For this review, take the finished solid that the model builds, in its own axes (mm). A direction names the side the tool comes from. Give positions to 0.01 mm unless a question says otherwise; leave off trailing zeros. Loops run counter-clockwise (first coordinate to the right, second up) from the corner with the lowest first, then second, coordinate; pieces in that order, holes last. Notation, with made-up numbers: (65, 4.5) - (119, 4.5) arc R13 cw to (119, 19.5) - close; hole circle Ø5 at (88.25, 14.5). An arc over 180 degrees is marked (long way). Use CSV: the item, a comma, the result in double quotes. Start each with the question number.
1. For faces 5 (the cylindrical face through (41.251, 19.965, 1.521)), 6 (the cylindrical face through (-43.94, 46.8, 4.14)), 7 (the flat face through (-49.85, 43.11, 11.9)), list the 3-axis set-ups (+Z, -Z, +X, -X, +Y, -Y) from which the entire face can be reached by the end or side of a thin tool; tool diameter is ignored.
2. Take a section at B-B on z = 10. State how many separate pieces and enclosed holes the cut face has, plus the area to 3 significant figures.
3. Wall thickness on line 1 (Y direction, x = 0, z = 2); line 2 (Z direction, x = 76, y = 23); line 3 (X direction, y = 18.5, z = 13.5): over which ranges is each line inside the solid? List them lowest first.
4. Mouldability with a two-part tool opening along Y and no side actions: class faces 1 (the flat face through (-47, 44, 24)), 2 (the cylindrical face through (40.62, 42.5, 1.52)), 3 (the flat face through (2.524, 54.735, 12.673)), 4 (the cylindrical face through (-51.829, 43.084, 4.141)) as pulls with the +Y half, pulls with the -Y half, needs draft (parallel to the pull), parting line crosses it, or undercut.
5. Take a section at A-A on y = 34. Give the boundary of the cut face in (x, z), plus the area to 3 significant figures.
6. Take a section at C-C on x = 20.5. Give the boundary of the cut face in (y, z), plus the area to 3 significant figures.
7. For pin 1 (3 mm diameter, centred on x = 50.5, z = 17, fed in from -Y); pin 2 (0.9 mm diameter, centred on x = -60, z = 1.5, fed in from +Y); pin 3 (3.5 mm diameter, centred on x = 14.5, z = 2, fed in from +Y), all flat-tipped, find the tip position at first contact; note any pin that passes through.
```python
from build123d import *

# Parameters (mm, degrees)
BOSS_EXTRUDE1_DEPTH = 3
BOSS_EXTRUDE2_DEPTH = 21
SKETCH3_R           = 1.5875
CUT_EXTRUDE1_DEPTH  = 111.972114009
FILLET3_R           = 4
FILLET4_R           = 4


with BuildPart() as part:
    # Sketch1 → Boss-Extrude1 (new body)
    with BuildSketch(Plane.XY):
        Polygon((0, 57.752828942), (48.814800356, 46.930848245), (88.482467371, 16.492776794), (92.403575887, 13.484004407), (84.489061716, 13.484004407), (-84.489061716, 13.484004407), (-92.403575887, 13.484004407), (-88.482467371, 16.492776794), (-48.814800356, 46.930848245), align=None)
    extrude(amount=BOSS_EXTRUDE1_DEPTH)

    # Sketch2 → Boss-Extrude2 (add)
    with BuildSketch(Plane.XY.offset(3)):
        Polygon((-45.368475451, 47.694880082), (-48.814800356, 46.930848245), (-51.615337647, 44.781920401), (-50.154310218, 42.877872384), (-49.138817942, 43.657087013), (-47.799542798, 41.911709664), (-48.815035074, 41.132495035), (-47.354007644, 39.228447018), (-45.784645761, 40.432660745), (-43.853398153, 40.860808032), (-44.372853227, 43.203918449), (-45.622512116, 42.926875744), (-46.098679267, 45.074726959), (-44.849020377, 45.351769665), align=None)
        Polygon((0, 57.752828942), (-3.446324905, 56.988797105), (-2.926869832, 54.645686688), (-1.677210943, 54.922729393), (-1.201043792, 52.774878178), (-2.450702681, 52.497835472), (-1.931247608, 50.154725055), (0, 50.582872342), (1.931247608, 50.154725055), (2.450702681, 52.497835472), (1.201043792, 52.774878178), (1.677210943, 54.922729393), (2.926869832, 54.645686688), (3.446324905, 56.988797105), align=None)
        Polygon((-84.22090265, 16.737656622), (-85.681930079, 18.641704639), (-92.403575887, 13.484004407), (-81.724287495, 13.484004407), (-82.881627506, 14.992279274), (-83.897119781, 14.213064644), (-85.236394925, 15.958441993), align=None)
        Polygon((48.814800356, 46.930848245), (45.368475451, 47.694880082), (44.849020377, 45.351769665), (46.098679267, 45.074726959), (45.622512116, 42.926875744), (44.372853227, 43.203918449), (43.853398153, 40.860808032), (45.784645761, 40.432660745), (47.354007644, 39.228447018), (48.815035074, 41.132495035), (47.799542798, 41.911709664), (49.138817942, 43.657087013), (50.154310218, 42.877872384), (51.615337647, 44.781920401), align=None)
        Polygon((82.881627506, 14.992279274), (81.724287495, 13.484004407), (92.403575887, 13.484004407), (85.681930079, 18.641704639), (84.22090265, 16.737656622), (85.236394925, 15.958441993), (83.897119781, 14.213064644), align=None)
    extrude(amount=BOSS_EXTRUDE2_DEPTH)

    # Sketch3 → Cut-Extrude1 (cut, through all)
    with BuildSketch(Plane.XY.offset(3)):
        with Locations((0, 18.484004407)):
            Circle(SKETCH3_R)
        with Locations((0, 38.484004407)):
            Circle(SKETCH3_R)
        with BuildLine():
            Line((-70.662620138, 23.864064428), (-52.799548931, 37.570881053))
            ThreePointArc((-52.799548931, 37.570881053), (-50.323945802, 38.119709054), (-48.312232144, 36.576066872))
            Line((-48.312232144, 36.576066872), (-41.176915041, 22.869250246))
            ThreePointArc((-41.176915041, 22.869250246), (-41.273211929, 19.927684632), (-43.837947541, 18.484004407))
            Line((-43.837947541, 18.484004407), (-68.836335851, 18.484004407))
            ThreePointArc((-68.836335851, 18.484004407), (-71.677126239, 20.519686011), (-70.662620138, 23.864064428))
        make_face()
        with BuildLine():
            Line((-32.570257259, 20.33595411), (-40.714847995, 39.998735523))
            ThreePointArc((-40.714847995, 39.998735523), (-40.604241897, 42.53203166), (-38.592528239, 44.075673842))
            Line((-38.592528239, 44.075673842), (-9.178295063, 50.596652343))
            ThreePointArc((-9.178295063, 50.596652343), (-6.713094257, 50.055770329), (-5.533087617, 47.82477219))
            Line((-5.533087617, 47.82477219), (-4.17050626, 21.825171068))
            ThreePointArc((-4.17050626, 21.825171068), (-5.038091405, 19.473478629), (-7.341155033, 18.484004407))
            Line((-7.341155033, 18.484004407), (-29.798618662, 18.484004407))
            ThreePointArc((-29.798618662, 18.484004407), (-31.465329361, 18.98959557), (-32.570257259, 20.33595411))
        make_face()
        with BuildLine():
            Line((7.341155033, 18.484004407), (29.798618662, 18.484004407))
            ThreePointArc((29.798618662, 18.484004407), (31.465329361, 18.98959557), (32.570257259, 20.33595411))
            Line((32.570257259, 20.33595411), (40.714847995, 39.998735523))
            ThreePointArc((40.714847995, 39.998735523), (40.604241897, 42.53203166), (38.592528239, 44.075673842))
            Line((38.592528239, 44.075673842), (9.178295063, 50.596652343))
            ThreePointArc((9.178295063, 50.596652343), (6.713094257, 50.055770329), (5.533087617, 47.82477219))
            Line((5.533087617, 47.82477219), (4.17050626, 21.825171068))
            ThreePointArc((4.17050626, 21.825171068), (5.038091405, 19.473478629), (7.341155033, 18.484004407))
        make_face()
        with BuildLine():
            Line((43.837947541, 18.484004407), (68.836335851, 18.484004407))
            ThreePointArc((68.836335851, 18.484004407), (71.677126239, 20.519686011), (70.662620138, 23.864064428))
            Line((70.662620138, 23.864064428), (52.799548931, 37.570881053))
            ThreePointArc((52.799548931, 37.570881053), (50.323945802, 38.119709054), (48.312232144, 36.576066872))
            Line((48.312232144, 36.576066872), (41.176915041, 22.869250246))
            ThreePointArc((41.176915041, 22.869250246), (41.273211929, 19.927684632), (43.837947541, 18.484004407))
        make_face()
    extrude(amount=-CUT_EXTRUDE1_DEPTH, mode=Mode.SUBTRACT)

    # Fillet3
    fillet3_edges = [part.edges().sort_by_distance(p)[0] for p in [
        (-84.951416365, 17.689680631, 3),
    ]]
    fillet(fillet3_edges, radius=FILLET3_R)

    # Fillet4
    fillet4_edges = [part.edges().sort_by_distance(p)[0] for p in [
        (84.951416365, 17.689680631, 3),
        (50.884823932, 43.829896392, 3),
        (45.108747914, 46.523324874, 3),
        (3.186597368, 55.817241896, 3),
        (-3.186597368, 55.817241896, 3),
        (-45.108747914, 46.523324874, 3),
        (-82.302957501, 14.23814184, 3),
        (-50.884823932, 43.829896392, 3),
        (82.302957501, 14.23814184, 3),
    ]]
    fillet(fillet4_edges, radius=FILLET4_R)


solid = part.part
```
Check result:
1,face 5,"+Z, -Z"
1,face 6,"+Z, +Y"
1,face 7,"+Z, -Y"
2,separate pieces,"5"
2,enclosed holes,"0"
2,area,"148 mm²"
3,line 1,"y = 13.48 to 16.9, 20.07 to 36.9, 40.07 to 57.75"
3,line 2,"z = 0 to 3"
3,line 3,"x = -85.87 to -85.57, 85.57 to 85.87"
4,face 1,"needs draft"
4,face 2,"undercut"
4,face 3,"undercut"
4,face 4,"pulls with the -Y half"
5,outline,"(-65.67, 0) - (-57.45, 0) - (-57.45, 3) - (-65.67, 3) - close; (-46.97, 0) - (-38.23, 0) - (-38.23, 3) - (-46.97, 3) - close; (-4.81, 0) - (4.81, 0) - (4.81, 3) - (-4.81, 3) - close; (38.23, 0) - (46.97, 0) - (46.97, 3) - (38.23, 3) - close; (57.45, 0) - (65.67, 0) - (65.67, 3) - (57.45, 3) - close"
5,area,"131 mm²"
6,outline,"(13.48, 0) - (18.48, 0) - (18.48, 3) - (13.48, 3) - close; (48.09, 0) - (53.21, 0) - (53.21, 3) - (48.09, 3) - close"
6,area,"30.4 mm²"
7,pin 1,"stops at y = 42.88"
7,pin 2,"stops at y = 38.69"
7,pin 3,"stops at y = 54.93"
